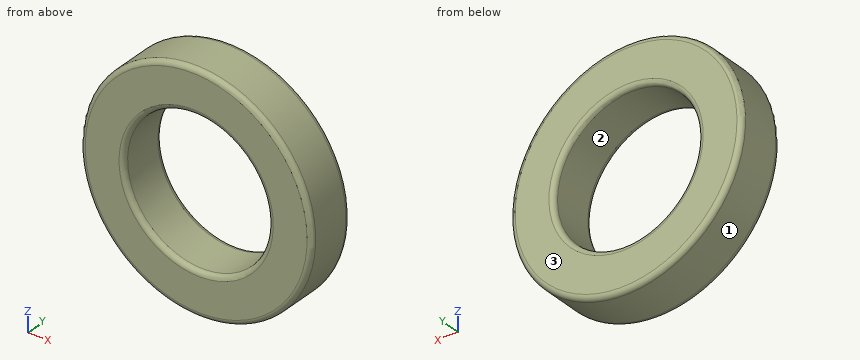
```python
from build123d import *


with BuildPart() as part:
    # Sketch1 → Revolve1 (revolve)
    with BuildSketch(Plane(origin=(0, 0, 0), x_dir=(-1, 0, 0), z_dir=(0, 0, -1)), mode=Mode.PRIVATE) as revolve1_sk:
        with BuildLine():
            Line((-12, -0.5), (-12, -4.5))
            ThreePointArc((-12, -4.5), (-11.853553391, -4.853553391), (-11.5, -5))
            Line((-11.5, -5), (-8, -5))
            ThreePointArc((-8, -5), (-7.646446609, -4.853553391), (-7.5, -4.5))
            Line((-7.5, -4.5), (-7.5, -0.5))
            ThreePointArc((-7.5, -0.5), (-7.646446609, -0.146446609), (-8, 0))
            Line((-8, 0), (-11.5, 0))
            ThreePointArc((-11.5, 0), (-11.853553391, -0.146446609), (-12, -0.5))
        make_face()
    revolve(revolve1_sk.sketch.rotate(Axis((0, -5, 0), (0, 1, 0)), 270), axis=Axis((0, -5, 0), (0, 1, 0)))


solid = part.part
```
The listing builds one solid part. Answer for the finished solid, in the listing's coordinates (mm). Face numbers are marked on the shaded views. Coordinates: 2 decimals unless noted, no trailing zeros. Write each loop counter-clockwise with the first axis right and the second up, starting at its lowest first coordinate (ties: lowest second). Pieces come first, ordered by that corner, then holes. Notation, with made-up numbers: M 78.25,7 L 117.25,7 A15 ccw 117.25,29 Z; hole C 70,-1.75 d10. An arc over 180 degrees is marked long. Use a Markdown table: item, result. Add a question column.
1. Straight lines are drawn through the part: line 1 along X through (y, z) = (-2.25, 0); line 2 along X through (y, z) = (-3.7, -1); line 3 along Z through (x, y) = (-0.5, -0.9). For each, find the intervals that lie inside material, in ascending order. Write a range as [from, to].
2. For a pull along X with two mould halves and no side action, classify the marked faces 1, 2 and 3 as +X half, -X half, draft (parallel to the pull), parting line (faces both ways), or undercut.
3. Given P1, Ø2, axis at x = 2, z = 5, coming from the +Y side; P2, Ø3, axis at x = -9.5, z = -7, coming from the +Y side, each flat-ended and moving along its own axis, determine where each tip first touches the part or whether it passes through.
4. Section C-C (y = -2.85) is taken. Give the vertices of the cut face in (x, z), plus the area to 3 significant figures.
5. Section A-A (z = 0) is taken. Give the vertices of the cut face in (x, y).
6. Section B-B (x = 0) is taken. Give the vertices of the cut face in (y, z).
Data:
| question | item | result |
|---|---|---|
| 1 | line 1 | x = [-12, -7.5], [7.5, 12] |
| 1 | line 2 | x = [-11.96, -7.43], [7.43, 11.96] |
| 1 | line 3 | z = [-11.99, -7.48], [7.48, 11.99] |
| 2 | face 1 | parting line |
| 2 | face 2 | undercut |
| 2 | face 3 | draft |
| 3 | P1 | passes through |
| 3 | P2 | stops at y = 0 |
| 4 | outline | C 0,0 d24; hole C 0,0 d15 |
| 4 | area | 276 mm2 |
| 5 | outline | M -12,-4.5 A0.5 ccw -11.5,-5 L -8,-5 A0.5 ccw -7.5,-4.5 L -7.5,-0.5 A0.5 ccw -8,0 L -11.5,0 A0.5 ccw -12,-0.5 Z; M 7.5,-4.5 A0.5 ccw 8,-5 L 11.5,-5 A0.5 ccw 12,-4.5 L 12,-0.5 A0.5 ccw 11.5,0 L 8,0 A0.5 ccw 7.5,-0.5 Z |
| 6 | outline | M -5,-11.5 A0.5 ccw -4.5,-12 L -0.5,-12 A0.5 ccw 0,-11.5 L 0,-8 A0.5 ccw -0.5,-7.5 L -4.5,-7.5 A0.5 ccw -5,-8 Z; M -5,8 A0.5 ccw -4.5,7.5 L -0.5,7.5 A0.5 ccw 0,8 L 0,11.5 A0.5 ccw -0.5,12 L -4.5,12 A0.5 ccw -5,11.5 Z |
